Can you work these out from the model? Positions are in its coordinate system, mm. A direction names the side the tool comes from. Give positions to 0.01 mm unless a question says otherwise; leave off trailing zeros. Order: outer loops, then holes, each group sorted by start corner. A loop starts at its lowest first (then second) coordinate and runs counter-clockwise, first axis right, second up. Notation, with made-up numbers: (79, -14.75) - (94, -14.75) arc R20 cw to (94, -10.75) - close; hole circle Ø4 at (55, 60.25). An arc over 180 degrees is marked (long way). Answer as CSV lines item,"result".
```python
from build123d import *

# Parameters (mm, degrees)
F1_DEPTH  = 101.6
F2_W      = 38.1
F2_H      = 25.4
F3_DEPTH  = 38.1
F4_W      = 38.1
F4_H      = 25.4
F5_DEPTH  = 38.1
F6_R      = 6.35
F7_W      = 50.8
F7_H      = 25.4
F8_DEPTH  = 101.601
F9_R      = 6.35
F10_W     = 101.6
F10_H     = 101.6
F11_DEPTH = 76.2
F13_DEPTH = 76.2
F15_START = -25.4
F15_DEPTH = 25.4


with BuildPart() as f1:
    # F0 (on Front) → F1 (new body)
    with BuildSketch(Plane.XZ):
        Polygon((0, 25.4), (0, 0), (101.6, 0), (101.6, 25.4), (139.7, 25.4), (139.7, 50.8), (-38.1, 50.8), (-38.1, 25.4), align=None)
    extrude(amount=F1_DEPTH)

    # F2 (on face) → F3 (cut)
    with BuildSketch(Plane.YZ.offset(139.7)):
        with Locations((-50.8, 38.1)):
            Rectangle(F2_W, F2_H)
    extrude(amount=-F3_DEPTH, mode=Mode.SUBTRACT)

    # F4 (on face) → F5 (cut)
    with BuildSketch(Plane(origin=(-38.1, 0, 0), x_dir=(0, -1, 0), z_dir=(-1, 0, 0))):
        with Locations((50.8, 38.1)):
            Rectangle(F4_W, F4_H)
    extrude(amount=-F5_DEPTH, mode=Mode.SUBTRACT)

    # F6
    f6_edges = [f1.edges().sort_by_distance(p)[0] for p in [
        (139.7, -101.6, 38.1),
        (139.7, 0, 38.1),
        (-38.1, -101.6, 38.1),
        (-38.1, 0, 38.1),
    ]]
    fillet(f6_edges, radius=F6_R)

    # F7 (on face) → F8 (cut, through all)
    with BuildSketch(Plane.XZ.offset(101.6)):
        with Locations((50.8, 12.7)):
            Rectangle(F7_W, F7_H)
    extrude(amount=-F8_DEPTH, mode=Mode.SUBTRACT)

    # F9
    f9_edges = [f1.edges().sort_by_distance(p)[0] for p in [
        (25.4, -50.8, 25.4),
        (76.2, -50.8, 25.4),
    ]]
    fillet(f9_edges, radius=F9_R)

    # F10 (on face) → F11 (join)
    with BuildSketch(Plane.XY.offset(50.8)):
        with Locations((38.1, -50.8)):
            Rectangle(F10_W, F10_H)
    extrude(amount=F11_DEPTH)

    # F12 (on face) → F13 (cut)
    with BuildSketch(Plane.XY.offset(127)):
        Polygon((88.9, 0), (38.1, -101.6), (88.9, -101.6), align=None)
        Polygon((38.1, -101.6), (-12.7, 0), (-12.7, -101.6), align=None)
    extrude(amount=-F13_DEPTH, mode=Mode.SUBTRACT)

    # F14 (on face) → F15 (cut)
    with BuildSketch(Plane.XY.offset(127).offset(F15_START)):
        Polygon((63.5, -50.8), (12.7, -50.8), (38.1, -101.6), align=None)
    extrude(amount=-F15_DEPTH, mode=Mode.SUBTRACT)


solid = f1.part
```
1) I want a section at D-D on y = -41.5. Write out the boundary of the cut face in (x, z).
Answer block:
outline,"(0, 0) - (25.4, 0) - (25.4, 19.05) arc R6.35 cw to (31.75, 25.4) - (69.85, 25.4) arc R6.35 cw to (76.2, 19.05) - (76.2, 0) - (101.6, 0) - (101.6, 50.8) - (68.15, 50.8) - (68.15, 127) - (8.05, 127) - (8.05, 50.8) - (0, 50.8) - close"
2) If we mould it in two halves opening along Z, with no side actions, what happens to faces 4 (the flat face through (50, -101.6, 36)), 5 (the flat face through (38, -70, 101.6)), 6 (the flat face through (51, -52, 25.4))? For each: +Z half, -Z half, draft (parallel to the pull), parting line (faces both ways), or undercut.
Answer block:
face 4,"draft"
face 5,"undercut"
face 6,"-Z half"
3) Which directions (+Z, -Z, +X, -X, +Y, -Y) give clear straight access to the entire face, cutting with the end or side of a thin tool? Please do faces 1 (the flat face through (120, -16, 25.4)), 2 (the flat face through (38, -50.8, 89)), 3 (the cylindrical face through (27.31, -50.09, 23.59)).
Answer block:
face 1,"-Z, +X, +Y, -Y"
face 2,"+X, -X, -Y"
face 3,"-Z, +Y, -Y"
4) I want a section at C-C on z = 46.5. Write out the boundary of the cut face in (x, y), plus the area to 3 significant figures.
Answer block:
outline,"(-38.1, -95.25) arc R6.35 ccw to (-31.75, -101.6) - (133.35, -101.6) arc R6.35 ccw to (139.7, -95.25) - (139.7, -69.85) - (101.6, -69.85) - (101.6, -31.75) - (139.7, -31.75) - (139.7, -6.35) arc R6.35 ccw to (133.35, 0) - (-31.75, 0) arc R6.35 ccw to (-38.1, -6.35) - (-38.1, -31.75) - (0, -31.75) - (0, -69.85) - (-38.1, -69.85) - close"
area,"15,100 mm2"
5) I'm going to push flat-ended pins straight in: P1, Ø9.5, axis at y = -75.5, z = 14, coming from the +X side; P2, Ø4, axis at y = -42.5, z = 105.5, coming from the -X side; P3, Ø5, axis at x = 31, y = -57.5, coming from the -Z side; P4, Ø8, axis at x = 107.5, z = 24, coming from the -Y side. Where does each tip first touch, or does it pass through?
Answer block:
P1,"x = 101.6"
P2,"x = 7.55"
P3,"z = 24.51"
P4,"y = -101.6"
6) I need wall thicknesses on line 1 along Z through (x, y) = (36, -85); line 2 along X through (y, z) = (-27, 12); line 3 along Y through (x, z) = (104, 37.5). Which ranges of each line are inside material? Lowest first, please. Write a range as [from, to].
Answer block:
line 1,"[25.4, 76.2], [101.6, 127]"
line 2,"[0, 25.4], [76.2, 101.6]"
line 3,"[-101.6, -69.85], [-31.75, 0]"
7) I want a section at A-A on x = 108.5. Write out the boundary of the cut face in (y, z).
Answer block:
outline,"(-101.6, 25.4) - (-69.85, 25.4) - (-69.85, 50.8) - (-101.6, 50.8) - close; (-31.75, 25.4) - (0, 25.4) - (0, 50.8) - (-31.75, 50.8) - close"
8) I want a section at B-B on y = -53. Write out the boundary of the cut face in (x, z), plus the area to 3 significant figures.
Answer block:
outline,"(0, 0) - (25.4, 0) - (25.4, 19.05) arc R6.35 cw to (31.75, 25.4) - (69.85, 25.4) arc R6.35 cw to (76.2, 19.05) - (76.2, 0) - (101.6, 0) - (101.6, 50.8) - (62.4, 50.8) - (62.4, 76.2) - (13.8, 76.2) - (13.8, 50.8) - (0, 50.8) - close; (13.8, 101.6) - (62.4, 101.6) - (62.4, 127) - (13.8, 127) - close"
area,"6,360 mm2"
